Input: part model. Units: mm. Frame: model coordinates. A direction names the side the tool comes from. Give positions to 0.01 mm unless a question says otherwise; leave off trailing zeros. Order: outer loops, then holes, each group sorted by start corner. A loop starts at its lowest first (then second) coordinate and runs counter-clockwise, first axis right, second up. Notation, with made-up numbers: (13, -18) - (31, -18) arc R23 cw to (31, 6) - close; hole circle Ø7 at (-19.5, 28.25). An arc over 180 degrees is marked (long way). Answer in a Markdown table with one row per item. Add a question column.
1. Access query for faces 4 (the face through (0, 31, 363)), 5 (the face through (1.588, 14, 363)). Directions: +Z, -Z, +X, -X, +Y, -Y. A direction counts if a zero-diameter tool reaches every point of the face in a straight line with its end or side. Return the directions, or none.
2. Section query B-B on z = 210.5. Return loops of the section in (x, y), and give its area (3 significant figures).
3. Section query A-A on y = 41.5. Return loops of the section in (x, z), and give its area (3 significant figures).
4. Contact query for a flat-ended pin moving along its axis: pin 1 (4 mm diameter, centred on x = 12.7, z = 63.5, fed in from -Y). Output: stop coordinate, or through.
5. Mould query, pull axis Y, two halves, no side actions, for faces 1 (the face through (25.4, 19, 363)), 2 (the face through (13, 50.8, 363)), 3 (the face through (13, 49.212, 363)). Classes: released by +Y, released by -Y, zero draft, split by the parting line, or undercut.
6. Ray query, line 1 (Z direction, x = 20.75, y = 49.85); line 2 (X direction, y = 50, z = 647); line 3 (X direction, y = 0.4, z = 88.9). Return the intervals inside material, ascending. Write a range as [from, to].
Autodesk Inventor part; units mm, degrees
ref_plane "YZ Plane" through (0, 0, 0) normal (1, 0, 0) x (0, 1, 0)
ref_plane "XZ Plane" through (0, 0, 0) normal (0, 1, 0) x (-1, 0, 0)
ref_plane "XY Plane" through (0, 0, 0) normal (0, 0, 1) x (1, 0, 0)
sketch "Sketch1" plane through (0, 0, 0) normal (0, 0, 1) x (1, 0, 0)
  line L0 (0, 0) -> (25.4, 0)
  line L1 (25.4, 0) -> (25.4, 50.8)
  line L2 (25.4, 50.8) -> (0, 50.8)
  line L3 (0, 50.8) -> (0, 0)
  line L4 (1.5875, 49.2125) -> (23.8125, 49.2125)
  line L5 (23.8125, 49.2125) -> (23.8125, 1.5875)
  line L6 (23.8125, 1.5875) -> (1.5875, 1.5875)
  line L7 (1.5875, 1.5875) -> (1.5875, 49.2125)
  dimension "d0" = 25.4
  dimension "d1" = 50.8
  dimension "d2" = 1.5875
extrude "Extrusion1" add sketch "Sketch1" along normal blind 736.6
sketch "Sketch4" plane through (0, 50.8, 0) normal (0, 1, 0) x (1, 0, 0)
  line L0 (1.5875, 0) -> (23.8125, 0) construction
  line L1 (12.7, 0) -> (12.7, -12.7) construction
  line L2 (12.7, -12.7) -> (12.7, -38.1) construction
  line L3 (12.7, -38.1) -> (12.7, -63.5) construction
  line L4 (0, 0) -> (0, -736.6) construction
  line L5 (0, -368.3) -> (25.4, -368.3) construction
  line L6 (25.4, 0) -> (25.4, -736.6) construction
  circle A0 centre (12.7, -12.7) radius 2.5797
  circle A1 centre (12.7, -38.1) radius 2.5797
  circle A2 centre (12.7, -63.5) radius 2.5797
  circle A3 centre (12.7, -723.9) radius 2.5797
  circle A4 centre (12.7, -698.5) radius 2.5797
  circle A5 centre (12.7, -673.1) radius 2.5797
  dimension "d15" = 12.7
  dimension "d16" = 25.4
  dimension "d17" = 25.4
  dimension "d18" = 5.1594
extrude "Extrusion4" cut sketch "Sketch4" against normal blind 152.4
sketch "Sketch5" plane through (25.4, 0, 0) normal (1, 0, 0) x (0, 0, -1)
  line L0 (0, 50.8) -> (-736.6, 50.8) construction
  line L1 (-368.3, 50.8) -> (-368.3, 25.4) construction
  circle A0 centre (-368.3, 25.4) radius 7.493
  point P0 (0, 0)
  dimension "d21" = 25.4
  dimension "d22" = 14.986
extrude "Extrusion5" cut sketch "Sketch5" against normal blind 25.4
sketch "Sketch6" plane through (0, 50.8, 0) normal (0, 1, 0) x (1, 0, 0)
  line L0 (0, 0) -> (25.4, 0) construction
  line L1 (25.4, 0) -> (25.4, -736.6) construction
  line L2 (0, -88.9) -> (4.75, -88.9) construction
  line L3 (4.75, -88.9) -> (20.75, -88.9) construction
  line L4 (20.75, -88.9) -> (20.75, -102.4) construction
  line L5 (20.75, -102.4) -> (4.75, -102.4) construction
  circle A0 centre (4.75, -88.9) radius 2.3
  circle A1 centre (20.75, -88.9) radius 2.3
  circle A2 centre (20.75, -102.4) radius 2.3
  circle A3 centre (4.75, -102.4) radius 2.3
  line L6 (0, 0) -> (0, -368.3) construction
  line L7 (0, 0) -> (0, -736.6) construction
  line L8 (0, -368.3) -> (25.4, -368.3) construction
  line L9 (0, -647.7) -> (4.75, -647.7) construction
  line L10 (4.75, -647.7) -> (20.75, -647.7) construction
  line L11 (20.75, -647.7) -> (20.75, -634.2) construction
  line L12 (20.75, -634.2) -> (4.75, -634.2) construction
  circle A4 centre (4.75, -647.7) radius 2.3
  circle A5 centre (20.75, -647.7) radius 2.3
  circle A6 centre (20.75, -634.2) radius 2.3
  circle A7 centre (4.75, -634.2) radius 2.3
  dimension "d26" = 88.9
  dimension "d28" = 4.75
  dimension "d29" = 16
  dimension "d30" = 13.5
  dimension "d31" = 4.6
  dimension "d33" = 368.3
extrude "Extrusion6" cut sketch "Sketch6" against normal blind 277.8125
properties part number "1x1 29in"
Answer:
| question | item | result |
|---|---|---|
| 1 | face 4 | +Z, -Z, -X, +Y, -Y |
| 1 | face 5 | +Z, -Z |
| 2 | outline | (0, 0) - (25.4, 0) - (25.4, 50.8) - (0, 50.8) - close; hole (1.59, 1.59) - (23.81, 1.59) - (23.81, 49.21) - (1.59, 49.21) - close |
| 2 | area | 232 mm² |
| 3 | outline | (0, 0) - (1.59, 0) - (1.59, 736.6) - (0, 736.6) - close; (23.81, 0) - (25.4, 0) - (25.4, 736.6) - (23.81, 736.6) - close |
| 3 | area | 2,340 mm² |
| 4 | pin 1 | passes through |
| 5 | face 1 | zero draft |
| 5 | face 2 | released by +Y |
| 5 | face 3 | undercut |
| 6 | line 1 | z = [0, 86.6], [91.2, 100.1], [104.7, 631.9], [636.5, 645.4], [650, 736.6] |
| 6 | line 2 | x = [0, 2.56], [6.94, 18.56], [22.94, 25.4] |
| 6 | line 3 | x = [0, 2.45], [7.05, 18.45], [23.05, 25.4] |
